Work out the finished part from the listing and answer in its coordinate system (mm). A direction names the side the tool comes from. Coordinates: 2 decimals unless noted, no trailing zeros. Loops run counter-clockwise (first coordinate to the right, second up) from the corner with the lowest first, then second, coordinate; pieces in that order, holes last. Notation, with made-up numbers: (14.5, 34.5) - (31.5, 34.5) arc R13 ccw to (31.5, 46.5) - close; hole circle Ø1 at (10, -0.75). An arc over 180 degrees is marked (long way). Write each question's results on one line, items separated by ' | '. Start each with the question number.
Item 1: Each of these flat-tipped pins is pushed along its axis until it touches: pin 1 Ø6 at (x, z) = (-296, 163.5) entering from -Y; pin 2 Ø1 at (x, z) = (-112.5, -5.5) entering from -Y; pin 3 Ø5 at (x, y) = (-121.5, -298.5) entering from +Z. Where does it stop, or does it pass through?
Item 2: Section B-B, the plane x = -232.5 is taken. Count the separate pieces of the cut face and the enclosed holes in it, plus the area to 3 significant figures.
Item 3: For a pull along Z with two mould halves and no side action, classify faces 1 (the face through (-259.321, -158.356, 5.704)), 2 (the face through (-49, -20, -2)), 3 (the face through (-79, 0, -3)) as +Z half, -Z half, draft (parallel to the pull), parting line (faces both ways), or undercut.
Item 4: A tool of negligible diameter and unlimited length cuts with its end or side. For faces 4 (the face through (-221.82, -129.53, 4.88)), 5 (the face through (-288.224, -306.651, 6.339)), 6 (the face through (0, -299, -24)), from which of +Z, -Z, +X, -X, +Y, -Y can it reach the whole face along a straight path? Write none if from no direction.
Item 5: Section C-C, the plane y = -61 is taken. Write down the section's boundary in (x, z) (3 decimals).
Item 6: Consider probe 1 along Y at (x, z) = (-52, 139) (1 decimal); probe 2 along Z at (x, y) = (-57, -88); probe 3 along Y at (x, z) = (-69, -81) (3 decimals). Determine where each line is inside the solid, lowest interval first. Write a range as [from, to].
Item 7: Section A-A, the plane y = -184.5 is taken. Write down the section's boundary in (x, z) (1 decimal).
Autodesk Inventor part; units mm, degrees
ref_plane "YZ Plane" through (0, 0, 0) normal (1, 0, 0) x (0, 1, 0)
ref_plane "XZ Plane" through (0, 0, 0) normal (0, 1, 0) x (-1, 0, 0)
ref_plane "XY Plane" through (0, 0, 0) normal (0, 0, 1) x (1, 0, 0)
sketch "スケッチ1" plane through (0, 0, 0) normal (1, 0, 0) x (0, 1, 0)
  line L0 (0, 0) -> (0, 200)
  line L1 (0, 200) -> (-400, 350)
  arc A0 (-400, 350) -> (-486.675, 0) centre (263.325, 0) ccw
  line L2 (-668.2907, 0) -> (453.5942, 0)
  line L3 (0, 0) -> (-20, 0)
  line L4 (-20, 0) -> (-20, 180.8)
  line L5 (-20, 180.8) -> (-381.217, 316.2564)
  arc A1 (-381.217, 316.2564) -> (-451.675, 0) centre (293.325, 0) ccw
  line L6 (-451.675, 0) -> (-486.675, 0)
  dimension "d0" = 200
  dimension "d1" = 400
  dimension "d2" = 750
  dimension "d3" = 350
  dimension "d9" = 20
  dimension "d10" = 25
  dimension "d11" = 30
  dimension "d12" = 35
revolve "回転2" add sketch "スケッチ1" angle 180 about axis through (0, -10, 0) along (0, -1, 0) contours L2 L4 L5 A1 A0 L1 L0
sketch "スケッチ2" plane through (0, 263.325, 0) normal (1, 0, 0) x (0, 0, -1)
  line L0 (-284.5531, -560) -> (0, -560)
  line L1 (0, -560) -> (0, -565)
  line L2 (0, -565) -> (-286.4281, -565)
  line L3 (-286.4281, -565) -> (-284.5531, -560)
  line L4 (-316.2564, -644.542) -> (-180.8, -283.325)
  arc A0 (-316.2564, -644.542) -> (0, -715) centre (0, 30) ccw
  line L5 (0, -906) -> (0, 186)
  point P0 (0, -263.325)
  dimension "d14" = 5
  dimension "d15" = 150
revolve "回転3" add sketch "スケッチ2" angle 180 about axis through (0, -10, 0) along (0, -1, 0) contours L0 L1 L2 L3
sketch "スケッチ3" plane through (0, 263.325, 0) normal (1, 0, 0) x (0, 0, -1)
  line L0 (-180.8, -283.325) -> (180.8, -283.325)
  line L1 (-284.5531, -560) -> (284.5531, -560)
  line L2 (-130, -283.325) -> (-130, -560)
  line L3 (-125, -283.325) -> (-125, -560)
  line L4 (0, -847.335) -> (0, -165.9899)
  line L5 (-130, -283.325) -> (-125, -283.325)
  line L6 (-130, -560) -> (-125, -560)
  line L7 (-284.5531, -560) -> (284.5531, -560)
  point P0 (0, -263.325)
  dimension "d17" = 5
  dimension "d18" = 125
revolve "回転4" add sketch "スケッチ3" angle 180 about axis through (0, -10, 0) along (0, -1, 0) contours L0 L3 L1 L2
properties part number "hakoooo"
Answer key:
1) pin 1: stops at y = -407.62 | pin 2: stops at y = -478.24 | pin 3: stops at z = 288.76
2) separate pieces: 1 | enclosed holes: 2 | area: 52,500 mm^2
3) face 1: parting line | face 2: undercut | face 3: draft
4) face 4: none | face 5: +X | face 6: +Z, -Z, +X, +Y, -Y
5) outline: (0, -222.875) - (0, -196.175) arc R196.175 cw to (0, 196.175) - (0, 222.875) arc R222.875 ccw to start; (0, -130) - (0, -125) arc R125 cw to (0, 125) - (0, 130) arc R130 ccw to start
6) probe 1: y = [-471.8, -436.7], [-301.7, -296.7], [-20, 0] | probe 2: z = [-225.92, -198.27], [-116.84, -111.25], [111.25, 116.84], [198.27, 225.92] | probe 3: y = [-479.089, -444.037], [-301.675, -296.675], [-20, 0]
7) outline: (0, -269.2) - (0, -242.5) arc R242.5 cw to (0, 242.5) - (0, 269.2) arc R269.2 ccw to start; (0, -130) - (0, -125) arc R125 cw to (0, 125) - (0, 130) arc R130 ccw to start
